Here's how the part is built. I have some questions about the finished solid (model axes, mm). Face numbers are marked on the shaded views. A direction names the side the tool comes from. Round coordinates to 2 decimals unless told otherwise and drop trailing zeros. Write each loop counter-clockwise with the first axis right and the second up, starting at its lowest first coordinate (ties: lowest second). Pieces come first, ordered by that corner, then holes. Notation, with made-up numbers: (61.25, -17.75) -> (78.25, -17.75) arc R3 cw to (78.25, -12.75) -> close; hole circle Ø10 at (43, 77.25). An arc over 180 degrees is marked (long way). Put each result on its own line as item: value. Start each with the question number.
1) We'd pull the mould along X, two halves only. Please class the marked faces 1, 2 and 3: released by +X, released by -X, zero draft, split by the parting line, or undercut.
2) Will these pins go through, and if not, where does the flat tip stop? P1, Ø1, axis at x = 11, z = 10.5, coming from the +Y side; P2, Ø1.1, axis at x = 11.5, z = 11.35, coming from the -Y side; P3, Ø3, axis at x = 3.5, y = 9.5, coming from the +Z side.
3) I want a section at B-B, the plane z = 16.25. List the corners of the cut face in (x, y) for me, then the cut area to 3 significant figures.
4) If I drill on line 1 along X through (y, z) = (0.8, 11.35); line 2 along Z through (x, y) = (7.5, 3.5); line 3 along X through (y, z) = (5, 17.5), over which ranges is the centre line in solid material (lowest first)? Write a range as [from, to].
5) I want a section at A-A, the plane y = 2. List the corners of the cut face in (x, z) for me, then the cut area to 3 significant figures.
6) I want a section at D-D, the plane y = 4. List the corners of the cut face in (x, z) for me, then the cut area to 3 significant figures.
7) I want a section at C-C, the plane x = 3.5. List the corners of the cut face in (y, z) for me.
8) Which directions (+Z, -Z, +X, -X, +Y, -Y) give clear straight access to the entire face, cutting with the end or side of a thin tool? Please do the marked faces 4 and 5.
from build123d import *

# Parameters (mm, degrees)
SKETCH_1_W           = 15
SKETCH_1_H           = 32.4
EXTRUDE_1_DEPTH      = 12.75
SKETCH_1_3_R         = 6.25
SKETCH_1_3_R_2       = 3
CUT_EXTRUDE_1_DEPTH  = 38.912036347
SKETCH_2_OUTSIDE_W   = 24.582
SKETCH_2_OUTSIDE_H   = 41.982
SKETCH_2_OUTSIDE_W_2 = 15
SKETCH_2_OUTSIDE_H_2 = 21.35
CUT_EXTRUDE_2_DEPTH  = 38.912036347
SKETCH_3_R           = 0.6
CUT_EXTRUDE_3_DEPTH  = 3
SKETCH_4_R           = 0.6
CUT_EXTRUDE_4_DEPTH  = 3


with BuildPart() as part:
    # Sketch 1 → Extrude 1 (new body)
    with BuildSketch(Plane(origin=(0, 0, 0), x_dir=(1, 0, 0), z_dir=(0, 1, 0))):
        with Locations((7.5, -16.2)):
            Rectangle(SKETCH_1_W, SKETCH_1_H)
    extrude(amount=EXTRUDE_1_DEPTH)

    # Sketch 1_3 → Cut-Extrude 1 (cut, through all)
    with BuildSketch(Plane(origin=(0, 0, 0), x_dir=(1, 0, 0), z_dir=(0, 1, 0))):
        with Locations((7.5, -21.35)):
            Circle(SKETCH_1_3_R)
        with Locations((7.5, -15.6)):
            Circle(SKETCH_1_3_R_2)
    extrude(amount=CUT_EXTRUDE_1_DEPTH, mode=Mode.SUBTRACT)

    # Sketch 2 outside → Cut-Extrude 2 (cut, through all)
    with BuildSketch(Plane(origin=(0, 12.75, 0), x_dir=(1, 0, 0), z_dir=(0, 1, 0))):
        with Locations((7.5, -16.2)):
            Rectangle(SKETCH_2_OUTSIDE_W, SKETCH_2_OUTSIDE_H)
        with Locations((7.5, -10.675)):
            Rectangle(SKETCH_2_OUTSIDE_W_2, SKETCH_2_OUTSIDE_H_2, mode=Mode.SUBTRACT)
    extrude(amount=-CUT_EXTRUDE_2_DEPTH, mode=Mode.SUBTRACT)

    # Sketch 3 → Cut-Extrude 3 (cut)
    with BuildSketch(Plane.XZ):
        with Locations(Location((3.5, 11.35, 0), (0, 0, 270))):
            Circle(SKETCH_3_R)
        with Locations(Location((11.5, 11.35, 0), (0, 0, 270))):
            Circle(SKETCH_3_R)
    extrude(amount=-CUT_EXTRUDE_3_DEPTH, mode=Mode.SUBTRACT)

    # Sketch 4 → Cut-Extrude 4 (cut)
    with BuildSketch(Plane(origin=(0, 12.75, 0), x_dir=(1, 0, 0), z_dir=(0, 1, 0))):
        with Locations(Location((11.25, -10.675, 0), (0, 0, 270))):
            Circle(SKETCH_4_R)
        with Locations(Location((3.75, -10.675, 0), (0, 0, 270))):
            Circle(SKETCH_4_R)
    extrude(amount=-CUT_EXTRUDE_4_DEPTH, mode=Mode.SUBTRACT)


solid = part.part
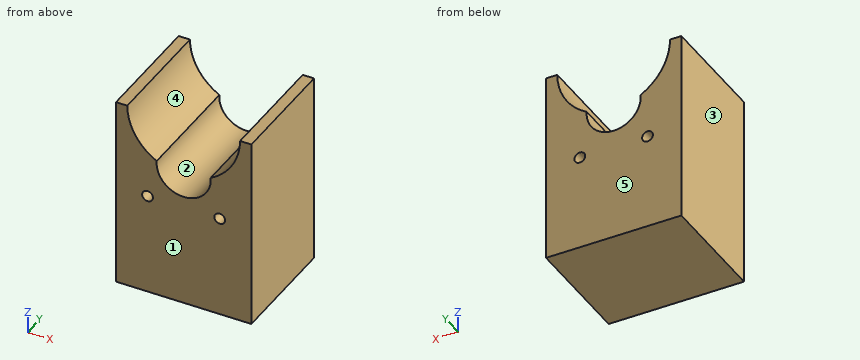
Findings:
1. face 1: zero draft
1. face 2: undercut
1. face 3: released by -X
2. P1: stops at y = 12.75
2. P2: stops at y = 3
2. P3: stops at z = 18.38
3. outline: (0, 0) -> (3.89, 0) -> (3.89, 12.75) -> (0, 12.75) -> close; (11.11, 0) -> (15, 0) -> (15, 12.75) -> (11.11, 12.75) -> close
3. area: 99.1 mm2
4. line 1: x = [0, 2.9], [4.1, 10.9], [12.1, 15]
4. line 2: z = [0, 12.6]
4. line 3: x = [0, 2.58], [12.42, 15]
5. outline: (0, 0) -> (15, 0) -> (15, 21.35) -> (13.75, 21.35) arc R6.25 cw to (10.49, 15.86) arc R3 cw (long way) to (4.51, 15.86) arc R6.25 cw to (1.25, 21.35) -> (0, 21.35) -> close; hole circle Ø1.2 at (3.5, 11.35); hole circle Ø1.2 at (11.5, 11.35)
5. area: 244 mm2
6. outline: (0, 0) -> (15, 0) -> (15, 21.35) -> (13.75, 21.35) arc R6.25 cw to (10.49, 15.86) arc R3 cw (long way) to (4.51, 15.86) arc R6.25 cw to (1.25, 21.35) -> (0, 21.35) -> close
6. area: 246 mm2
7. outline: (0, 0) -> (12.75, 0) -> (12.75, 10.13) -> (9.75, 10.13) -> (9.75, 11.22) -> (12.75, 11.22) -> (12.75, 16.55) -> (0, 16.55) -> (0, 11.95) -> (3, 11.95) -> (3, 10.75) -> (0, 10.75) -> close
8. face 4: +Z, +Y, -Y
8. face 5: +Z, -Z, +X, -X, +Y
